Job drawing, mm, ordinate dimensions from the low corner. One solid piece. A direction names the side the tool comes from. Round coordinates to 2 decimals unless told otherwise and drop trailing zeros. Loops run counter-clockwise (first coordinate to the right, second up) from the corner with the lowest first, then second, coordinate; pieces in that order, holes last. Notation, with made-up numbers: M 12,63.5 L 53,63.5 A26 cw 53,101.5 Z; hole C -3.75,2.25 d6. An arc over 180 degrees is marked long. Use one line per item in the form item = value.
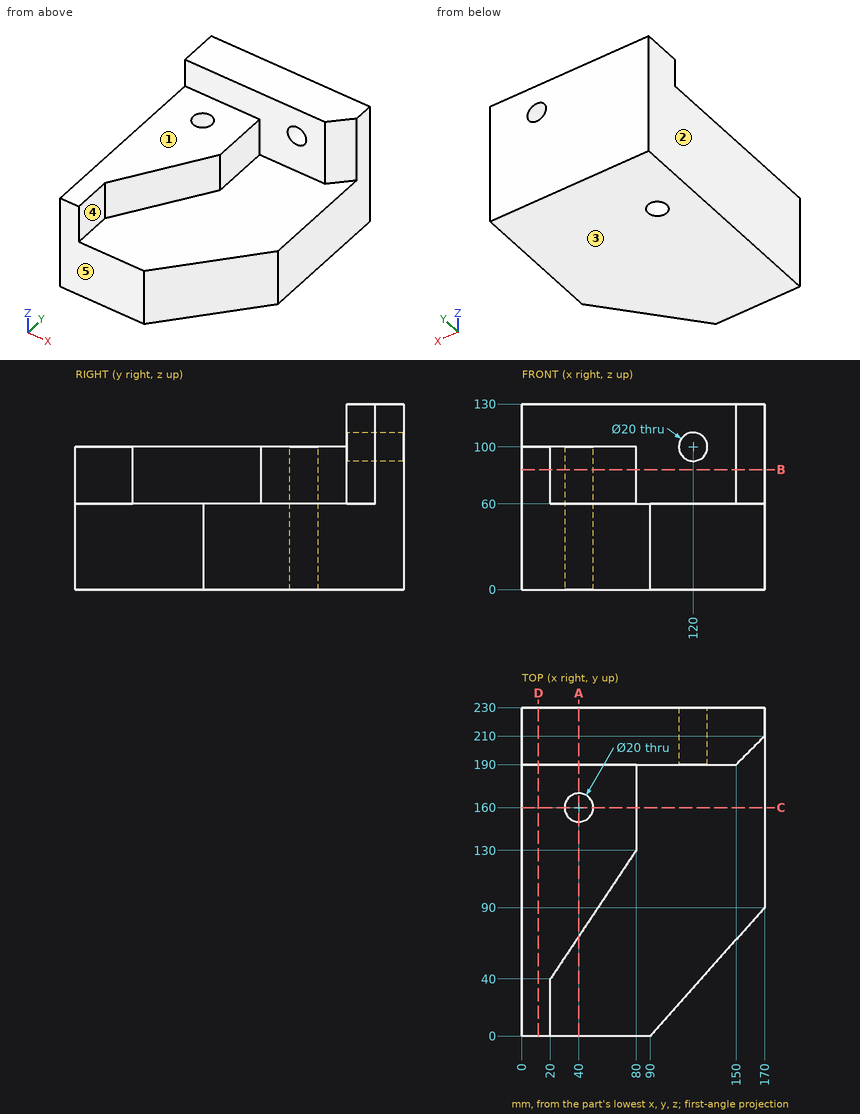
1. Tool access for the marked faces 4 and 5: list every direction of +Z, -Z, +X, -X, +Y, -Y with a clear straight run to the whole face (end or side of a thin tool).
Completed:
face_4 = +Z, +X, -Y
face_5 = +Z, -Z, +X, -X, -Y
2. Probe line 1 along Y through (x, z) = (40, 54); line 2 along Y through (x, z) = (135.5, 116.5); line 3 along Z through (x, y) = (106.5, 114). List the from-to ranges inside material, lowest first. Write a range as from..to.
Completed:
line_1 = 0..150, 170..230
line_2 = 190..230
line_3 = 0..60
3. Cut at D-D on x = 11.5. Write the cut outline in (y, z), and give its area (3 significant figures).
Completed:
outline = M 0,0 L 230,0 L 230,130 L 190,130 L 190,100 L 0,100 Z
area = 24,200 mm2
4. Cut at A-A on x = 40. Write the cut outline in (y, z), and give its area (3 significant figures).
Completed:
outline = M 0,0 L 150,0 L 150,100 L 70,100 L 70,60 L 0,60 Z; M 170,0 L 230,0 L 230,130 L 190,130 L 190,100 L 170,100 Z
area = 19,400 mm2
5. Drop flat-ended pins along their axis: P1, Ø18, axis at x = 40, y = 160, coming from the +Z side; P2, Ø12, axis at y = 169.5, z = 73, coming from the +X side; P3, Ø12, axis at y = 22.5, z = 79, coming from the +X side. Give the stop position or say it passes through.
Completed:
P1 = through
P2 = 80
P3 = 20
6. Cut at C-C on y = 160. Write the cut outline in (x, z), and give its area (3 significant figures).
Completed:
outline = M 0,0 L 30,0 L 30,100 L 0,100 Z; M 50,0 L 170,0 L 170,60 L 80,60 L 80,100 L 50,100 Z
area = 11,400 mm2
7. Pull direction Z, two halves, no side cores. Call the marked faces 1, 2 and 3: +Z half, -Z half, draft (parallel to the pull), parting line (faces both ways), or undercut.
Completed:
face_1 = +Z half
face_2 = draft
face_3 = -Z half
8. Cut at B-B on z = 84. Write the cut outline in (x, y).
Completed:
outline = M 0,0 L 20,0 L 20,40 L 80,130 L 80,190 L 150,190 L 170,210 L 170,230 L 0,230 Z; hole C 40,160 d20
